Build history of the part. All positions in model axes, mm. Face numbers are marked on the shaded views. Round coordinates to 2 decimals unless told otherwise and drop trailing zeros. Write each loop counter-clockwise with the first axis right and the second up, starting at its lowest first coordinate (ties: lowest second). Pieces come first, ordered by that corner, then holes.
Item 1: Drop flat-ended pins along their axis: pin 1 Ø5 at (x, z) = (7, 15) entering from +Y; pin 2 Ø1.5 at (x, z) = (-12, 4) entering from +Y; pin 3 Ø1 at (y, z) = (6, 13.5) entering from -X. Give the stop position or say it passes through.
Item 2: Mould opens along X. For the marked faces 1, 2 and 3 say: +X half, -X half, draft (parallel to the pull), parting line (faces both ways), or undercut.
Item 3: Band-saw the part on D-D, the plane z = 19.5. Write the cut outline in (x, y).
Item 4: Wall check: probe 1 along Z at (x, y) = (4.5, 17.5); probe 2 along X at (y, z) = (0.5, 19); probe 3 along X at (y, z) = (24.5, 18.75). Give the ranges that are in metal, low to high.
Item 5: Band-saw the part on C-C, the plane z = 11. Write the cut outline in (x, y).
```python
from build123d import *

# Parameters (mm, degrees)
F0_R     = 31.75
F1_DEPTH = 20.6375
F2_R     = 29.07284
F3_DEPTH = 3.175


# Not quite as in the source:
# - a fillet or chamfer that OpenCascade refuses, or shapes differently, is made with other operations: its cross-section is extruded or revolved along the edge and cut away or added


with BuildPart() as f1:
    # F0 (on Top) → F1 (new body)
    with BuildSketch(Plane.XY):
        Circle(F0_R)
    extrude(amount=F1_DEPTH)

    # F2 (on face) → F3 (cut)
    with BuildSketch(Plane.XY.offset(20.6375)):
        Circle(F2_R)
    extrude(amount=-F3_DEPTH, mode=Mode.SUBTRACT)

    # F4: fillet of radius 3.175 on 1 edges, made by hand

    # F4_s1 → F4_t2 (revolve, cut)
    with BuildSketch(Plane.XZ):
        with BuildLine():
            ThreePointArc((31.75, 17.5017735556), (30.9896704744, 19.5633243068), (29.07284, 20.6375))
            Line((29.07284, 20.6375), (31.75, 20.6375))
            Line((31.75, 20.6375), (31.75, 17.5017735556))
        make_face()
    revolve(axis=Axis((0, 0, 20.6375), (0, 0, 1)), mode=Mode.SUBTRACT)


solid = f1.part
```
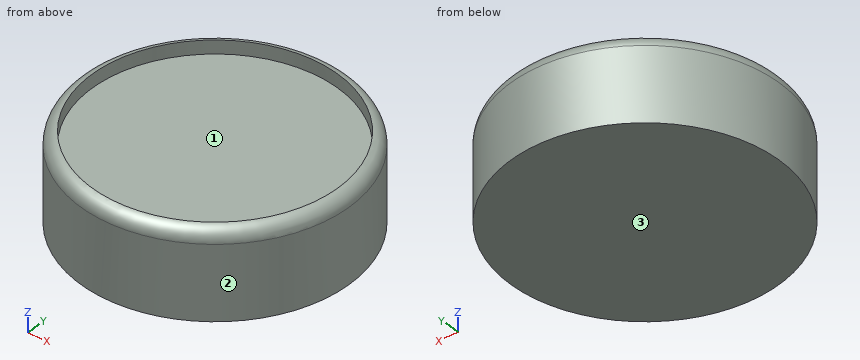
Results:
1. pin 1: stops at y = 31.43
1. pin 2: stops at y = 29.69
1. pin 3: stops at x = -31.27
2. face 1: undercut
2. face 2: parting line
2. face 3: draft
3. outline: circle Ø62.08 at (0, 0); hole circle Ø58.15 at (0, 0)
4. probe 1: z = 0 to 17.46
4. probe 2: x = -31.37 to -29.07, 29.07 to 31.37
4. probe 3: x = -19.79 to -15.65, 15.65 to 19.79
5. outline: circle Ø63.5 at (0, 0)
